Geometry: final body of the model. Coordinates: model frame, mm. A direction names the side the tool comes from. Coordinates: 2 decimals unless noted, no trailing zeros. Loops run counter-clockwise (first coordinate to the right, second up) from the corner with the lowest first, then second, coordinate; pieces in that order, holes last. Notation, with made-up numbers: (54, 30.25) - (59, 30.25) arc R6 ccw to (59, 40.25) - close; hole circle Ø7 at (60, 38). An arc over 180 degrees is marked (long way). Write each question's results on one line, items separated by ' | '. Start each with the question number.
from build123d import *

# Parameters (mm, degrees)
RESSALTO_EXTRUS_O1_DEPTH = 70
RESSALTO_EXTRUS_O2_REACH = 92.865


with BuildPart() as part:
    # Esboço1 → Ressalto-extrusão1 (new body)
    with BuildSketch(Plane.XY):
        Polygon((-46.166666667, -15.652777778), (33.833333333, 19.347222222), (33.833333333, -15.652777778), align=None)
    extrude(amount=RESSALTO_EXTRUS_O1_DEPTH)

    # Ressalto-extrusão2: up to this plane
    ressalto_extrus_o2_end = Plane(origin=(-46.166666667, -15.652777778, 70), z_dir=(0.4008188340197078, -0.9161573349021892, 0))
    # Esboço3 → Ressalto-extrusão2 (add, up to the surface)
    with BuildSketch(Plane.XZ.offset(15.652777778), mode=Mode.PRIVATE) as ressalto_extrus_o2_sk1:
        with BuildLine():
            Line((-10.666666667, 70), (-1.666666667, 70))
            Line((-1.666666667, 70), (-1.666666667, 75.846688069))
            ThreePointArc((-1.666666667, 75.846688069), (-6.166666667, 85.815315035), (-10.666666667, 75.846688069))
            Line((-10.666666667, 75.846688069), (-10.666666667, 70))
        make_face()
    ressalto_extrus_o2_tool1 = split(extrude(ressalto_extrus_o2_sk1.sketch, amount=-RESSALTO_EXTRUS_O2_REACH, mode=Mode.PRIVATE), bisect_by=ressalto_extrus_o2_end, keep=Keep.BOTH, mode=Mode.PRIVATE)
    add(ressalto_extrus_o2_tool1.solids().sort_by_distance((-6.166667, -15.652778, 77.842662))[0])


solid = part.part
1) Section query B-B on z = 54. Output: boundary loops of the cut face in (x, y).
2) Section query D-D on y = -5. Output: boundary loops of the cut face in (x, z).
3) Material intervals for line 1 (Z direction, x = 3, y = -6.5); line 2 (Y direction, x = -8, z = 57); line 3 (Y direction, x = 3, z = 26.5), sorted ascending. Write a range as [from, to].
4) Section query C-C on x = -23. Output: boundary loops of the cut face in (y, z).
5) Access query for faces 4 (the flat face through (33.833, 2, 35)), 5 (the flat face through (-1.667, -6, 73)), 6 (the flat face through (-10.667, -8, 73)). Directions: +Z, -Z, +X, -X, +Y, -Y. A direction counts if a zero-diameter tool reaches every point of the face in a straight line with its end or side. Return the directions, or none.
6) Section query A-A on y = -12.5. Output: boundary loops of the cut face in (x, z).
7) Pin query (flat end, axial travel): pin 1 Ø10 at (x, y) = (-37, -1.5) entering from +Z; pin 2 Ø10 at (y, z) = (7, 36.5) entering from -X; pin 3 Ø2 at (y, z) = (-10.5, 34.5) entering from -X; pin 4 Ø6.5 at (y, z) = (-8, 74) entering from +X. Return the tip coordinate at first contact, or that it passes through.
8) Pull-direction query (Z, two-part tool) for faces 1 (the flat face through (12, -6, 0)), 2 (the flat face through (-6.73, 1.6, 32.77)), 3 (the cylindrical face through (-3.073, -7.945, 84.956)); classes: released by +Z, released by -Z, zero draft, split by the parting line, or undercut.
Returned:
1) outline: (-46.17, -15.65) - (33.83, -15.65) - (33.83, 19.35) - close
2) outline: (-21.82, 0) - (33.83, 0) - (33.83, 70) - (-1.67, 70) - (-1.67, 75.85) arc R6 ccw (long way) to (-10.67, 75.85) - (-10.67, 70) - (-21.82, 70) - close
3) line 1: z = [0, 70] | line 2: y = [-15.65, 1.05] | line 3: y = [-15.65, 5.86]
4) outline: (-15.65, 0) - (-5.52, 0) - (-5.52, 70) - (-15.65, 70) - close
5) face 4: +Z, -Z, +X, +Y, -Y | face 5: +X, +Y, -Y | face 6: -X, +Y, -Y
6) outline: (-38.96, 0) - (33.83, 0) - (33.83, 70) - (-1.67, 70) - (-1.67, 75.85) arc R6 ccw (long way) to (-10.67, 75.85) - (-10.67, 70) - (-38.96, 70) - close
7) pin 1: passes through | pin 2: stops at x = -5.82 | pin 3: stops at x = -36.67 | pin 4: stops at x = -0.74
8) face 1: released by -Z | face 2: zero draft | face 3: undercut
